Print and shaded views of the part. All mm, measured from the part's lowest x, y and z. Give positions to 0.01 mm unless a question says otherwise; leave off trailing zeros. Loops run counter-clockwise (first coordinate to the right, second up) from the corner with the lowest first, then second, coordinate; pieces in that order, holes last. Notation, with made-up numbers: (46, 67.25) - (98, 67.25) arc R35 ccw to (98, 101.25) - close; hole circle Ø7 at (87.25, -25). An arc over 180 degrees is marked (long way). Return JSON: item names as keys, results as strings.
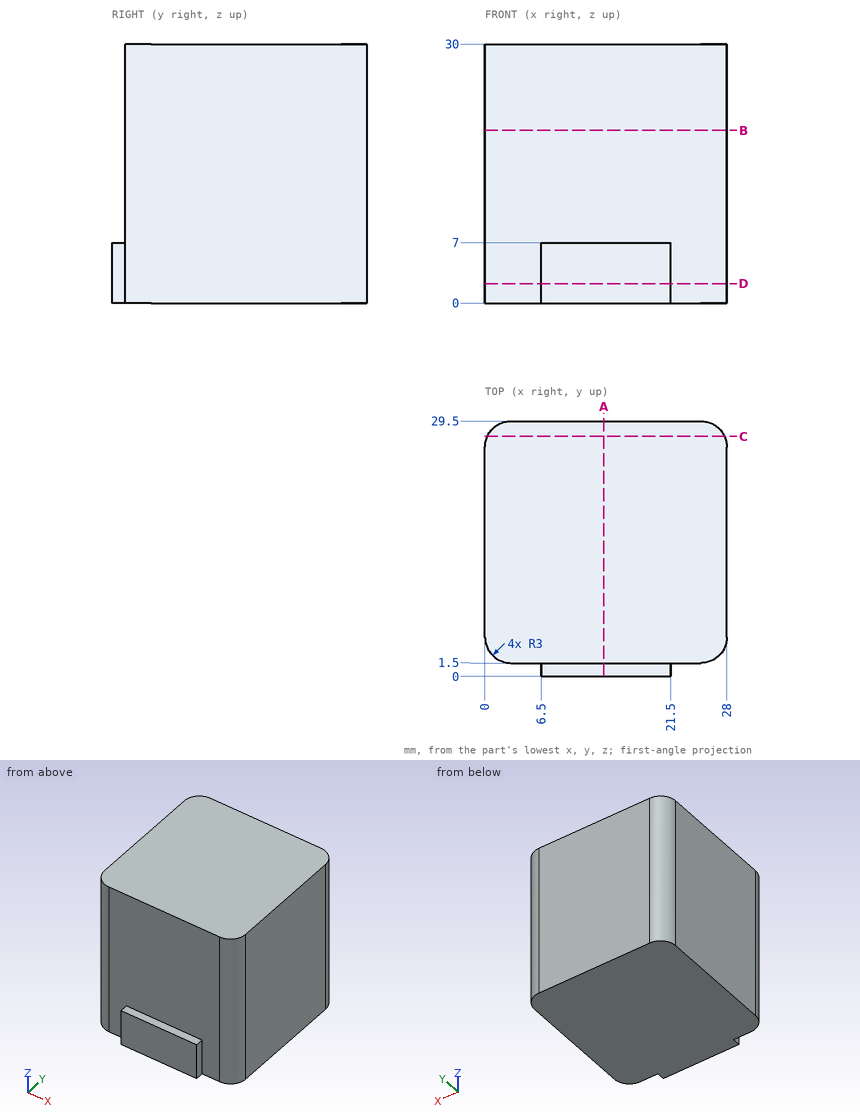
1. Cut at C-C, the plane y = 27.75. Write the cut outline in (x, z), plus the area to 3 significant figures.
Values follow:
{"outline": "(0.27, 0) - (27.73, 0) - (27.73, 30) - (0.27, 30) - close", "area": "824 mm²"}
2. Cut at D-D, the plane z = 2.25. Write the cut outline in (x, y), plus the area to 3 significant figures.
Values follow:
{"outline": "(0, 4.5) arc R3 ccw to (3, 1.5) - (6.5, 1.5) - (6.5, 0) - (21.5, 0) - (21.5, 1.5) - (25, 1.5) arc R3 ccw to (28, 4.5) - (28, 26.5) arc R3 ccw to (25, 29.5) - (3, 29.5) arc R3 ccw to (0, 26.5) - close", "area": "799 mm²"}
3. Cut at B-B, the plane z = 20. Write the cut outline in (x, y).
Values follow:
{"outline": "(0, 4.5) arc R3 ccw to (3, 1.5) - (25, 1.5) arc R3 ccw to (28, 4.5) - (28, 26.5) arc R3 ccw to (25, 29.5) - (3, 29.5) arc R3 ccw to (0, 26.5) - close"}
4. Cut at A-A, the plane x = 13.75. Write the cut outline in (y, z).
Values follow:
{"outline": "(0, 0) - (29.5, 0) - (29.5, 30) - (1.5, 30) - (1.5, 7) - (0, 7) - close"}
5. Drop a flat-ended pin along its axis: P1, Ø1.5, axis at x = 5, z = 25.5, coming from the -Y side. Give the stop position or say it passes through.
Values follow:
{"P1": "stops at y = 1.5"}
6. Drill centre lines: probe 1 along Y at (x, z) = (24, 26.25); probe 2 along X at (y, z) = (26.75, 28.5); probe 3 along X at (y, z) = (3, 14.5). Where is each one in solid material? Low to high.
Values follow:
{"probe 1": "y = 1.5 to 29.5", "probe 2": "x = 0.01 to 27.99", "probe 3": "x = 0.4 to 27.6"}
